```python
from build123d import *

# Parameters (mm, degrees)
F1_DEPTH = 100
F2_R     = 1


# Not quite as in the source:
# - ends of sketch curves that miss each other by under 0.0002 mm in the source are joined


with BuildPart() as f1:
    # F0 (on Front) → F1 (new body)
    with BuildSketch(Plane.XZ):
        Polygon((-75.7449854628, 50.6034867488), (-107.9829619636, 0), (-105.4527876261, -1.611898825), (-75.7449854628, 45.0200097587), (-43.5070133628, -5.5834700822), (-11.2690412628, 45.0200097587), (20.9689308372, -5.5834700822), (53.2069029372, 45.0200097587), (82.9147051006, -1.611898825), (85.444879438, 0), (53.2069029372, 50.6034867488), (20.9689264364, 0), (-11.2690412628, 50.6034867488), (-43.5070177636, 0), align=None)
    extrude(amount=F1_DEPTH)

    # F2
    f2_edges = [f1.edges().sort_by_distance(p)[0] for p in [
        (53.206903, -50, 50.603487),
        (-11.269041, -50, 50.603487),
        (-75.744985, -50, 50.603487),
        (-43.507013, -50, -5.58347),
        (20.968931, -50, -5.58347),
        (82.914705, -50, -1.611899),
        (-105.452788, -50, -1.611899),
        (-107.982962, -50, 0),
        (85.444879, -50, 0),
    ]]
    fillet(f2_edges, radius=F2_R)


solid = f1.part
```
Source: CAD feature listing. Evaluate the final solid. Frame: model axes, mm. A direction names the side the tool comes from. Give positions to 0.01 mm unless a question says otherwise; leave off trailing zeros. Write each loop counter-clockwise with the first axis right and the second up, starting at its lowest first coordinate (ties: lowest second). Pieces come first, ordered by that corner, then holes.
1. First-contact query: pin 1 (6 mm diameter, centred on y = -67.5, z = 1.5, fed in from -X); pin 2 (1.5 mm diameter, centred on x = -39, y = -38, fed in from +Z); pin 3 (1 mm diameter, centred on x = 55, y = -39.5, fed in from +Z); pin 4 (10 mm diameter, centred on x = 30, y = -75.5, fed in from -Z). Flat tips, straight axial feed; report the tip coordinate or a pass-through.
2. Section query C-C (x = -4.5). Return the cut outline in (y, z), then the cut area to 3 significant figures.
3. Material intervals for line 1 along X through (y, z) = (-34.5, 19.5); line 2 along X through (y, z) = (-47, 29); line 3 along X through (y, z) = (-65.5, 46.5), sorted ascending.
4. Access query for faces 1 (the face through (37.29, -49.3, 20.035)), 2 (the face through (-91.8, -49.3, 25.4)), 3 (the face through (-27.59, -49.3, 24.985)). Directions: +Z, -Z, +X, -X, +Y, -Y. A direction counts if a zero-diameter tool reaches every point of the face in a straight line with its end or side. Return the directions, or none.
5. Pull-direction query (X, two-part tool) for faces 4 (the face through (3, -100, 25)), 5 (the face through (69.695, -49.3, 24.722)), 6 (the face through (36.886, -49.3, 24.985)); classes: +X half, -X half, draft (parallel to the pull), parting line (faces both ways), or undercut.
6. Section query A-A (z = 28). Return the cut outline in (x, y) (3 decimals).
7. Section query D-D (z = 40). Return the cut outline in (x, y) (3 decimals).
8. Section query B-B (y = -26). Return the cut outline in (x, z).
Output values:
1. pin 1: stops at x = -107.6
1. pin 2: stops at z = 8.25
1. pin 3: stops at z = 48.57
1. pin 4: stops at z = 0.74
2. outline: (-100, 34.39) - (0, 34.39) - (0, 39.98) - (-100, 39.98) - close
2. area: 558 mm2
3. line 1: x = -95.56 to -92, -59.49 to -55.93, -31.08 to -27.53, 4.99 to 8.55, 33.39 to 36.95, 69.46 to 73.02
3. line 2: x = -89.51 to -85.95, -65.54 to -61.98, -25.03 to -21.47, -1.06 to 2.49, 39.44 to 43, 63.41 to 66.97
3. line 3: x = -78.36 to -73.13, -13.88 to -8.65, 50.59 to 55.82
4. face 1: -Z, +Y, -Y
4. face 2: +Z, -X, +Y, -Y
4. face 3: +Z, +Y, -Y
5. face 4: draft
5. face 5: +X half
5. face 6: undercut
6. outline: (-90.145, -100) - (-86.588, -100) - (-86.588, 0) - (-90.145, 0) - close; (-64.902, -100) - (-61.345, -100) - (-61.345, 0) - (-64.902, 0) - close; (-25.669, -100) - (-22.112, -100) - (-22.112, 0) - (-25.669, 0) - close; (-0.426, -100) - (3.131, -100) - (3.131, 0) - (-0.426, 0) - close; (38.807, -100) - (42.364, -100) - (42.364, 0) - (38.807, 0) - close; (64.05, -100) - (67.607, -100) - (67.607, 0) - (64.05, 0) - close
7. outline: (-82.5, -100) - (-78.943, -100) - (-78.943, 0) - (-82.5, 0) - close; (-72.547, -100) - (-68.99, -100) - (-68.99, 0) - (-72.547, 0) - close; (-18.024, -100) - (-14.467, -100) - (-14.467, 0) - (-18.024, 0) - close; (-8.071, -100) - (-4.514, -100) - (-4.514, 0) - (-8.071, 0) - close; (46.452, -100) - (50.009, -100) - (50.009, 0) - (46.452, 0) - close; (56.405, -100) - (59.962, -100) - (59.962, 0) - (56.405, 0) - close
8. outline: (-107.45, 0.84) arc R1 ccw to (-107.14, -0.54) - (-106.3, -1.07) arc R1 ccw to (-104.92, -0.77) - (-75.74, 45.02) - (-44.35, -4.26) arc R1 ccw to (-42.66, -4.26) - (-11.27, 45.02) - (20.13, -4.26) arc R1 ccw to (21.81, -4.26) - (53.21, 45.02) - (82.38, -0.77) arc R1 ccw to (83.76, -1.07) - (84.6, -0.54) arc R1 ccw to (84.91, 0.84) - (54.05, 49.28) arc R1 ccw to (52.36, 49.28) - (20.97, 0) - (-10.43, 49.28) arc R1 ccw to (-12.11, 49.28) - (-43.51, 0) - (-74.9, 49.28) arc R1 ccw to (-76.59, 49.28) - close
